Drawing for the job (mm, zero at the part's lowest x, y, z). A direction names the side the tool comes from. Give positions to 0.01 mm unless a question says otherwise; leave off trailing zeros. Write each loop counter-clockwise with the first axis right and the second up, starting at its lowest first coordinate (ties: lowest second). Pieces come first, ordered by that corner, then holes. Notation, with made-up numbers: M 26.5,-25 L 81.5,-25 A19 cw 81.5,-10 Z; hole C 88,-29.5 d8. An arc over 180 degrees is marked long. Answer as a JSON object with one key per item and string values. Group by question number.
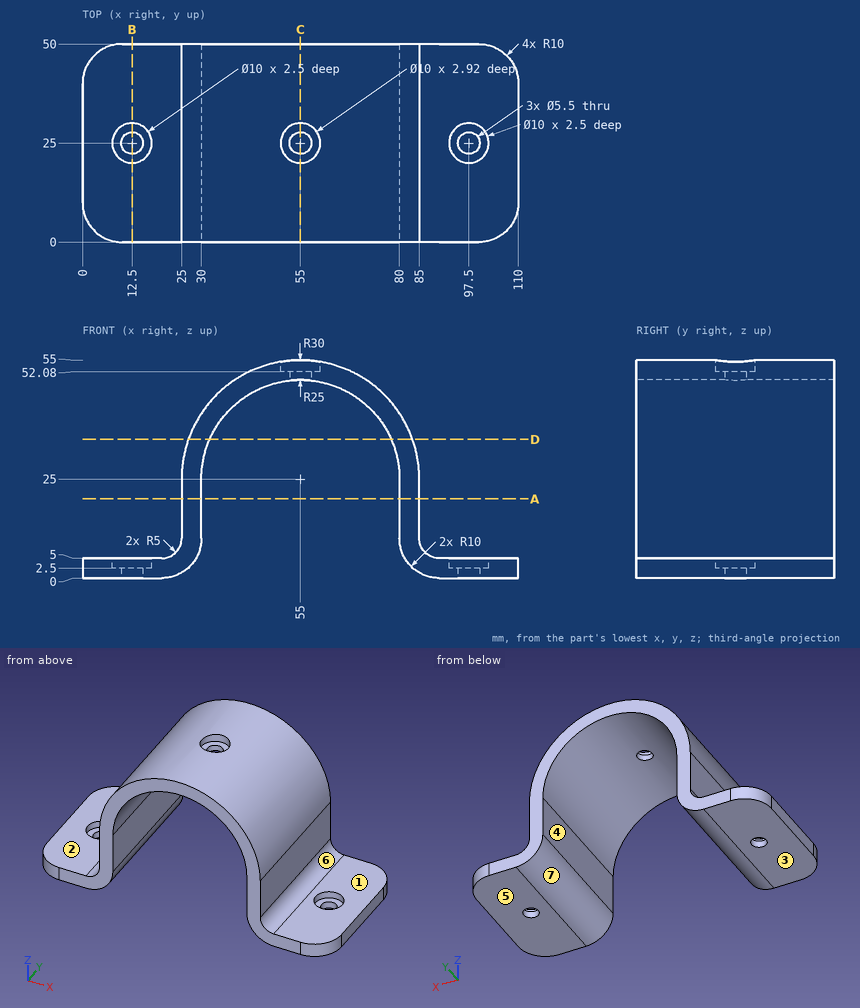
Q1. Slice it at C-C, the plane x = 55. Write the cut outline in (y, z).
Q2. Slice it at A-A, the plane z = 20. Write the cut outline in (x, y), then the cut area to 3 significant figures.
Q3. Slice it at D-D, the plane z = 35. Write the cut outline in (x, y) (1 decimal), then the cut area to 3 significant figures.
Q4. Slice it at B-B, the plane x = 12.5. Write the cut outline in (y, z).
Q5. 3-axis set-ups, long thin cutter, end or side, ignore diameter. For the marked faces 1, 2, 3 and 4: which of +Z, -Z, +X, -X, +Y, -Y reach the whole face in a straight line?
Q6. Drop flat-ended pins along their axis: P1, Ø10, axis at y = 45, z = 25, coming from the +X side; P2, Ø9, axis at x = 97.5, y = 25, coming from the -Z side; P3, Ø1.5, axis at y = 26, z = 33.5, coming from the +X side; P4, Ø3, axis at x = 75, y = 7, coming from the +Z side. Give the stop position or say it passes through.
Q7. Wall check: L1, parallel to X at y = 9, z = 22; L2, parallel to Y at x = 12.5, z = 1.75; L3, parallel to Y at x = 97, z = 3 (1 decimal). Give the ranges that are in metal, low to high.
Q8. Two-plate mould, pull along X, no slides. Class the marked faces 5, 6 and 7: +X half, -X half, draft (parallel to the pull), parting line (faces both ways), or undercut.
Solved:
{
 "1": {"outline": "M 0,50 L 22.25,50 L 22.25,52.08 L 20,52.08 L 20,55 L 0,55 Z; M 27.75,50 L 50,50 L 50,55 L 30,55 L 30,52.08 L 27.75,52.08 Z"},
 "2": {"outline": "M 25,0 L 30,0 L 30,50 L 25,50 Z; M 80,0 L 85,0 L 85,50 L 80,50 Z", "area": "500 mm²"},
 "3": {"outline": "M 26.7,0 L 32.1,0 L 32.1,50 L 26.7,50 Z; M 77.9,0 L 83.3,0 L 83.3,50 L 77.9,50 Z", "area": "537 mm²"},
 "4": {"outline": "M 0,0 L 22.25,0 L 22.25,2.5 L 20,2.5 L 20,5 L 0,5 Z; M 27.75,0 L 50,0 L 50,5 L 30,5 L 30,2.5 L 27.75,2.5 Z"},
 "5": {"face 1": "+Z, +X, +Y, -Y", "face 2": "+Z, -X, +Y, -Y", "face 3": "-Z, +X, -X, +Y, -Y", "face 4": "-Z, +Y, -Y"},
 "6": {"P1": "stops at x = 85", "P2": "stops at z = 0", "P3": "stops at x = 83.98", "P4": "stops at z = 48.62"},
 "7": {"L1": "x = 25 to 30, 80 to 85", "L2": "y = 0 to 22.25, 27.75 to 50", "L3": "y = 0 to 20, 30 to 50"},
 "8": {"face 5": "draft", "face 6": "+X half", "face 7": "undercut"}
}
